from build123d import *

# Parameters (mm, degrees)
ESBO_O_W                 = 111.5
ESBO_O_H                 = 55
RESSALTO_EXTRUS_O1_DEPTH = 22.5
CASCA3_T                 = 3
ESBO_O12_R               = 0.95
RESSALTO_EXTRUS_O2_DEPTH = 16
ESBO_O15_W               = 7.8
ESBO_O15_H               = 3.7
USB_DEPTH                = 3.9
ESBO_O16_R               = 1
RESSALTO_EXTRUS_O4_DEPTH = 2.81
ESBO_O17_R               = 0.74
RESSALTO_EXTRUS_O5_DEPTH = 12.6


with BuildPart() as part:
    # Esboço → Ressalto-extrusão1 (new body)
    with BuildSketch(Plane(origin=(0, 0, 0), x_dir=(1, 0, 0), z_dir=(0, 1, 0))):
        with Locations((-36.607366715, 20.784772609)):
            Rectangle(ESBO_O_W, ESBO_O_H)
    extrude(amount=RESSALTO_EXTRUS_O1_DEPTH)

    # Casca3
    casca3_openings = [part.faces().sort_by_distance(p)[0] for p in [
        (-36.607366715, 22.5, -20.784772609),
    ]]
    offset(amount=CASCA3_T, openings=casca3_openings, kind=Kind.INTERSECTION)

    # Esboço12 → Ressalto-extrusão2 (add)
    with BuildSketch(Plane(origin=(0, 0, 0), x_dir=(1, 0, 0), z_dir=(0, 1, 0))):
        with Locations(Location((-50.857366715, 43.784772609, 0), (0, 0, 270))):
            Circle(ESBO_O12_R)
        with Locations(Location((-88.857366715, 43.784772609, 0), (0, 0, 270))):
            Circle(ESBO_O12_R)
        with Locations(Location((-88.857366715, -2.215227391, 0), (0, 0, 270))):
            Circle(ESBO_O12_R)
        with Locations(Location((-50.857366715, -2.215227391, 0), (0, 0, 270))):
            Circle(ESBO_O12_R)
    extrude(amount=RESSALTO_EXTRUS_O2_DEPTH)

    # Esboço15 → usb (cut)
    with BuildSketch(Plane.XY.offset(9.715227391)):
        with Locations((-76.847366715, 6.44)):
            Rectangle(ESBO_O15_W, ESBO_O15_H)
    extrude(amount=-USB_DEPTH, mode=Mode.SUBTRACT)

    # Esboço16 → Ressalto-extrusão4 (add)
    with BuildSketch(Plane(origin=(0, 0, 0), x_dir=(1, 0, 0), z_dir=(0, 1, 0))):
        with Locations(Location((-84.517607583, 35.272111724, 0), (0, 0, 270))):
            Circle(ESBO_O16_R)
        with Locations(Location((-69.277607583, 35.272111724, 0), (0, 0, 270))):
            Circle(ESBO_O16_R)
        with Locations(Location((-69.277607583, -5.367888276, 0), (0, 0, 270))):
            Circle(ESBO_O16_R)
        with Locations(Location((-84.517607583, -5.367888276, 0), (0, 0, 270))):
            Circle(ESBO_O16_R)
    extrude(amount=RESSALTO_EXTRUS_O4_DEPTH)

    # Esboço17 → Ressalto-extrusão5 (add)
    with BuildSketch(Plane(origin=(0, 0, 0), x_dir=(1, 0, 0), z_dir=(0, 1, 0))):
        with Locations(Location((-30.447366715, 12.894772609, 0), (0, 0, 270))):
            Circle(ESBO_O17_R)
        with Locations(Location((4.912633285, 12.894772609, 0), (0, 0, 270))):
            Circle(ESBO_O17_R)
        with Locations(Location((4.912633285, -4.415227391, 0), (0, 0, 270))):
            Circle(ESBO_O17_R)
        with Locations(Location((-30.447366715, -4.415227391, 0), (0, 0, 270))):
            Circle(ESBO_O17_R)
    extrude(amount=RESSALTO_EXTRUS_O5_DEPTH)


solid = part.part
Geometry check sheet. Reference: the model listing, model coordinates, mm. A direction names the side the tool comes from. Give positions to 0.01 mm unless a question says otherwise; leave off trailing zeros. Order: outer loops, then holes, each group sorted by start corner. A loop starts at its lowest first (then second) coordinate and runs counter-clockwise, first axis right, second up. Notation, with made-up numbers: (-38, 75) - (-25, 75) arc R18 ccw to (-25, 98) - close; hole circle Ø11 at (36, 28.5). An arc over 180 degrees is marked (long way). Answer as a JSON object with one key per item and string values.
(1) Cross-section at B-B (z = -27.5). Record the cut outline in (x, y), then the cut area to 4 significant figures.
Report:
{"outline": "(-95.36, -3) - (22.14, -3) - (22.14, 22.5) - (19.14, 22.5) - (19.14, 0) - (-92.36, 0) - (-92.36, 22.5) - (-95.36, 22.5) - close", "area": "487.5 mm^2"}
(2) Material ranges on line 1 (X direction, y = 5.75, z = -37); line 2 (Z direction, x = -33, y = 4); line 3 (Y direction, x = -76.5, z = -35), recorded low to high.
Report:
{"line 1": "-95.36 to -92.36, 19.14 to 22.14", "line 2": "-51.28 to -48.28, 6.72 to 9.72", "line 3": "-3 to 0"}
(3) Draft check along Z on faces 1 (the flat face through (-37, 10, 9.715)), 2 (the flat face through (19.143, 11, -20)), 3 (the flat face through (-37, 0, -21)), 4 (the flat face through (-77, 4.59, 8)). Enter one of: released by +Z, released by -Z, zero draft, split by the parting line, or undercut.
Report:
{"face 1": "released by +Z", "face 2": "undercut", "face 3": "undercut", "face 4": "zero draft"}
(4) Depth check by flat-ended pin: pin 1 Ø0.6 at (x, z) = (-69.5, 5.5) entering from +Y; pin 2 Ø16.5 at (x, z) = (-38.5, -19.5) entering from +Y; pin 3 Ø1 at (x, z) = (-89, 2) entering from +Y. Enter the tip coordinate at first touch or a pass-through.
Report:
{"pin 1": "y = 2.81", "pin 2": "y = 0", "pin 3": "y = 16"}
(5) Cross-section at A-A (x = -9). Record the cut outline in (y, z), then the cut area to 3 significant figures.
Report:
{"outline": "(-3, -51.28) - (22.5, -51.28) - (22.5, -48.28) - (0, -48.28) - (0, 6.72) - (22.5, 6.72) - (22.5, 9.72) - (-3, 9.72) - close", "area": "318 mm^2"}
(6) Tool access check on faces 5 (the flat face through (-80.747, 6, 8)), 6 (the flat face through (-37, 10, -51.285)), 7 (the flat face through (-37, 11, -48.285)). Record the directions out of +Z, -Z, +X, -X, +Y, -Y that give a thin tool (end or side, any length) a straight path to the whole face; none if there is none.
Report:
{"face 5": "+Z", "face 6": "-Z, +X, -X, +Y, -Y", "face 7": "+Y"}
